```python
from build123d import *

# Parameters (mm, degrees)
BOSS_EXTRU_1_DEPTH      = 25
ESQUISSE2_R             = 1.5
BOSS_EXTRU_2_DEPTH      = 9.8
ESQUISSE3_W             = 31.176753694
ESQUISSE3_H             = 17.849543287
ENL_V_MAT_EXTRU_2_DEPTH = 0.2
ESQUISSE4_R             = 1.75
BOSS_EXTRU_3_DEPTH      = 5
ESQUISSE5_W             = 14.938362126
ESQUISSE5_H             = 3.694178454
ENL_V_MAT_EXTRU_3_DEPTH = 7.7
ESQUISSE6_W             = 7.972464104
ESQUISSE6_H             = 3.417362688
ENL_V_MAT_EXTRU_4_DEPTH = 7.7
BOSS_EXTRU_4_DEPTH      = 25
ESQUISSE8_R             = 1
ENL_V_MAT_EXTRU_5_DEPTH = 5


with BuildPart() as part:
    # Esquisse1 → Boss.-Extru.1 (new body)
    with BuildSketch(Plane(origin=(0, 0, 0), x_dir=(1, 0, 0), z_dir=(0, 1, 0))):
        with BuildLine():
            Line((17.783419244, -3), (21.484005679, -3))
            ThreePointArc((21.484005679, -3), (1.006821565, -23.012759245), (-21.25, -5))
            Line((-21.25, -5), (-17.5, -5))
            ThreePointArc((-17.5, -5), (1.009990899, -19.317966169), (17.783419244, -3))
        make_face()
    extrude(amount=-BOSS_EXTRU_1_DEPTH)

    # Esquisse2 → Boss.-Extru.2 (add)
    with BuildSketch(Plane(origin=(0, -17.5, 0), x_dir=(1, 0, 0), z_dir=(0, 1, 0))):
        with BuildLine():
            Line((-17.5, -5), (-25, -5))
            ThreePointArc((-25, -5), (-28.5, -1.5), (-25, 2))
            Line((-25, 2), (-17.219475506, 1.620843362))
            Line((-17.219475506, 1.620843362), (-17.5, -5))
        make_face()
        with Locations((-25, -1.5)):
            Circle(ESQUISSE2_R, mode=Mode.SUBTRACT)
    extrude(amount=BOSS_EXTRU_2_DEPTH)

    # Esquisse3 → Enlèv. mat.-Extru.2 (cut)
    with BuildSketch(Plane.XZ.offset(17.5)):
        with Locations((-26.283313767, -3.924771644)):
            Rectangle(ESQUISSE3_W, ESQUISSE3_H)
    extrude(amount=-ENL_V_MAT_EXTRU_2_DEPTH, mode=Mode.SUBTRACT)

    # Esquisse4 → Boss.-Extru.3 (add)
    with BuildSketch(Plane(origin=(0, 0, 3), x_dir=(-1, 0, 0), z_dir=(0, 0, -1))):
        with BuildLine():
            Line((-17.783419244, -17.5), (-24.935595774, -17.5))
            ThreePointArc((-24.935595774, -17.5), (-29.935595774, -12.5), (-24.935595774, -7.5))
            Line((-24.935595774, -7.5), (-17.783419244, -7.5))
            Line((-17.783419244, -7.5), (-17.783419244, -17.5))
        make_face()
        with Locations((-24.935595774, -12.5)):
            Circle(ESQUISSE4_R, mode=Mode.SUBTRACT)
    extrude(amount=-BOSS_EXTRU_3_DEPTH)

    # Esquisse5 → Enlèv. mat.-Extru.3 (cut)
    with BuildSketch(Plane(origin=(0, 0, 0), x_dir=(1, 0, 0), z_dir=(0, 1, 0))):
        with Locations((-16.074576592, -3.352910773)):
            Rectangle(ESQUISSE5_W, ESQUISSE5_H)
    extrude(amount=-ENL_V_MAT_EXTRU_3_DEPTH, mode=Mode.SUBTRACT)

    # Esquisse6 → Enlèv. mat.-Extru.4 (cut)
    with BuildSketch(Plane.XZ.offset(25)):
        with Locations((-19.148660485, 3.491318656)):
            Rectangle(ESQUISSE6_W, ESQUISSE6_H)
    extrude(amount=-ENL_V_MAT_EXTRU_4_DEPTH, mode=Mode.SUBTRACT)

    # Esquisse7 → Boss.-Extru.4 (add)
    with BuildSketch(Plane(origin=(0, 0, 0), x_dir=(1, 0, 0), z_dir=(0, 1, 0))):
        with BuildLine():
            Line((15, -11.169539803), (15, -23.036306554))
            Line((15, -23.036306554), (-15, -23.036306554))
            Line((-15, -23.036306554), (-15, -11.169539803))
            ThreePointArc((-15, -11.169539803), (0, -19.346568298), (15, -11.169539803))
        make_face()
    extrude(amount=-BOSS_EXTRU_4_DEPTH)

    # Esquisse8 → Enlèv. mat.-Extru.5 (cut)
    with BuildSketch(Plane.XY.offset(23.036306554)):
        with Locations((10.5, -22)):
            Circle(ESQUISSE8_R)
        with Locations((-10.5, -22)):
            Circle(ESQUISSE8_R)
        with Locations((10.5, -9.5)):
            Circle(ESQUISSE8_R)
        with Locations((-10.5, -9.5)):
            Circle(ESQUISSE8_R)
    extrude(amount=-ENL_V_MAT_EXTRU_5_DEPTH, mode=Mode.SUBTRACT)


solid = part.part
```
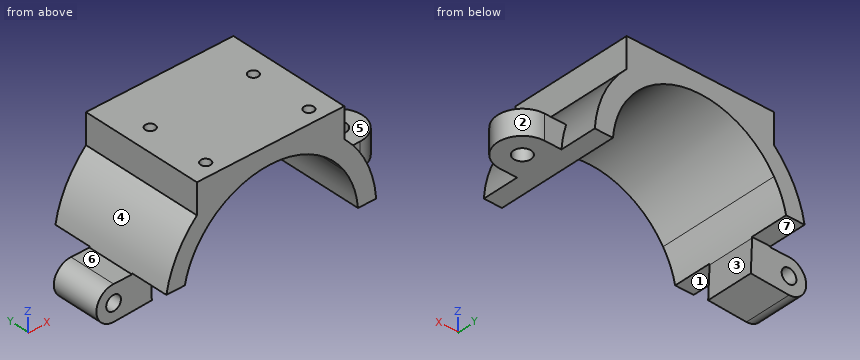
Model file for the job. Use its own axes, mm. Face numbers are marked on the shaded views. A direction names the side the tool comes from. Coordinates: 2 decimals unless noted, no trailing zeros. Loops run counter-clockwise (first coordinate to the right, second up) from the corner with the lowest first, then second, coordinate; pieces in that order, holes last. Notation, with made-up numbers: (9.25, 52) -> (62.25, 52) arc R16 cw to (62.25, 80) -> close; hole circle Ø6 at (63, 4). An arc over 180 degrees is marked (long way). Answer as a JSON object with one key per item and string values.
Q1. Cut at C-C (y = -22). List the corners of the cut face in (x, z), and give its area (3 significant figures).
Report:
{"outline": "(-21.22, 5.2) -> (-17.46, 5.2) arc R17.85 cw to (17.78, 3) -> (21.48, 3) arc R21.54 ccw to (15, 16.95) -> (15, 23.04) -> (11.5, 23.04) -> (11.5, 18.04) -> (9.5, 18.04) -> (9.5, 23.04) -> (-9.5, 23.04) -> (-9.5, 18.04) -> (-11.5, 18.04) -> (-11.5, 23.04) -> (-15, 23.04) -> (-15, 16.95) arc R21.54 ccw to start", "area": "246 mm2"}
Q2. Flat gauge pins, fed straight in: P1, Ø10, axis at y = -14, z = 16, coming from the -X side; P2, Ø1.6, axis at x = 10.5, y = -9.5, coming from the -Z side; P3, Ø2, axis at x = -18, y = -4.5, coming from the -Z side; P4, Ø2.5, axis at x = -25, z = 1.5, coming from the -Y side. Where does each tip first touch, or does it go through?
Report:
{"P1": "stops at x = -19.33", "P2": "stops at z = 15.31", "P3": "stops at z = 5.2", "P4": "passes through"}
Q3. Cut at B-B (x = 26). List the corners of the cut face in (y, z).
Report:
{"outline": "(-17.39, 3) -> (-13.89, 3) -> (-13.89, 8) -> (-17.39, 8) -> close; (-11.11, 3) -> (-7.61, 3) -> (-7.61, 8) -> (-11.11, 8) -> close"}
Q4. Probe probe 1 along Y at (x, z) = (-10.5, 20.7); probe 2 along Y at (x, z) = (25, 4.75); probe 3 along X at (y, z) = (-5, 20.5). List the from-to ranges inside material, lowest first.
Report:
{"probe 1": "y = -25 to -23, -21 to -10.5, -8.5 to 0", "probe 2": "y = -17.5 to -14.25, -10.75 to -7.5", "probe 3": "x = -15 to 15"}
Q5. Cut at D-D (z = 2.25). List the corners of the cut face in (x, y).
Report:
{"outline": "(-28.42, -17.3) -> (-26.3, -17.3) -> (-26.3, -7.7) -> (-28.42, -7.7) -> close; (-23.7, -17.3) -> (-17.38, -17.3) -> (-17.38, -7.7) -> (-23.7, -7.7) -> close"}
Q6. Cut at A-A (z = 21.25). List the corners of the cut face in (x, y).
Report:
{"outline": "(-15, -25) -> (15, -25) -> (15, 0) -> (-15, 0) -> close; hole circle Ø2 at (-10.5, -22); hole circle Ø2 at (-10.5, -9.5); hole circle Ø2 at (10.5, -22); hole circle Ø2 at (10.5, -9.5)"}
Q7. 3-axis set-ups, long thin cutter, end or side, ignore diameter. For the marked faces 5, 6 and 7: which of +Z, -Z, +X, -X, +Y, -Y reach the whole face in a straight line?
Report:
{"face 5": "+Z, +X, +Y, -Y", "face 6": "+Z, -X, +Y, -Y", "face 7": "-Z, -X, +Y"}
Q8. Pull direction X, two halves, no side cores. Call the marked faces 1, 2, 3 and 4: released by +X, released by -X, zero draft, split by the parting line, or undercut.
Report:
{"face 1": "zero draft", "face 2": "released by +X", "face 3": "undercut", "face 4": "released by -X"}
